Build history of the part. All positions in model axes, mm. Round coordinates to 2 decimals unless told otherwise and drop trailing zeros. Order: outer loops, then holes, each group sorted by start corner. A loop starts at its lowest first (then second) coordinate and runs counter-clockwise, first axis right, second up. Notation, with made-up numbers: M 12.5,63 L 24.5,63 A12 cw 24.5,71 Z; hole C 27,60 d5. An arc over 180 degrees is marked long. Use CSV: the item, a comma, the result in double quotes.
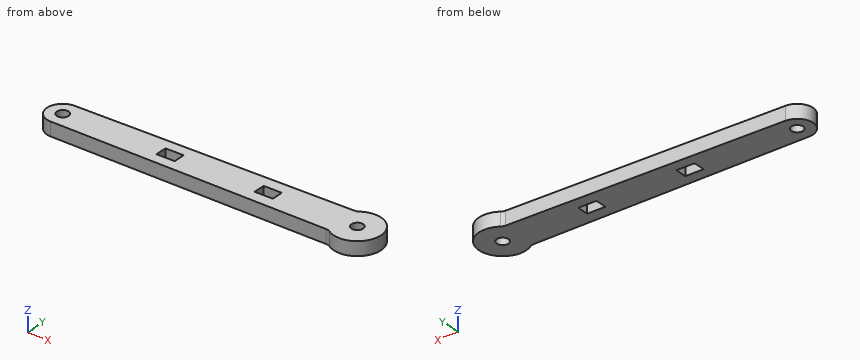
from build123d import *

# Parameters (mm, degrees)
SKETCH1_R           = 1.5
SKETCH1_W           = 4.635083662
SKETCH1_H           = 3
BOSS_EXTRUDE1_DEPTH = 3.5
FILLET1_R           = 2


with BuildPart() as part:
    # Sketch1 → Boss-Extrude1 (new body)
    with BuildSketch(Plane.XY):
        with BuildLine():
            Line((-75.039443802, 3.999805519), (-3.725751189, 4.703060501))
            ThreePointArc((-3.725751189, 4.703060501), (6, 0), (-3.725751189, -4.703060501))
            Line((-3.725751189, -4.703060501), (-75.039443802, -3.999805519))
            ThreePointArc((-75.039443802, -3.999805519), (-79, 0), (-75.039443802, 3.999805519))
        make_face()
        with Locations((-75, 0)):
            Circle(SKETCH1_R, mode=Mode.SUBTRACT)
        Circle(SKETCH1_R, mode=Mode.SUBTRACT)
        with Locations((-47.682458169, 0)):
            Rectangle(SKETCH1_W, SKETCH1_H, mode=Mode.SUBTRACT)
        with Locations((-22.682458169, 0)):
            Rectangle(SKETCH1_W, SKETCH1_H, mode=Mode.SUBTRACT)
    extrude(amount=BOSS_EXTRUDE1_DEPTH)

    # Fillet1
    fillet1_edges = [part.edges().sort_by_distance(p)[0] for p in [
        (-3.725751189, 4.703060501, 1.75),
        (-3.725751189, -4.703060501, 1.75),
    ]]
    fillet(fillet1_edges, radius=FILLET1_R)


solid = part.part
(1) Cut at B-B, the plane x = 0. Give the cut face in (y, z).
Answer block:
outline,"M -6,0 L -1.5,0 L -1.5,3.5 L -6,3.5 Z; M 1.5,0 L 6,0 L 6,3.5 L 1.5,3.5 Z"
(2) Drop flat-ended pins along their axis: pin 1 (1.8 mm diameter, centred on x = -23.5, z = 1, fed in from -Y); pin 2 (1.5 mm diameter, centred on x = -65.5, z = 2, fed in from +Y); pin 3 (2 mm diameter, centred on y = 2, z = 2.5, fed in from -X). Give the stop position or say it passes through.
Answer block:
pin 1,"stops at y = -4.52"
pin 2,"stops at y = 4.1"
pin 3,"stops at x = -78.87"
(3) Cut at C-C, the plane z = 2.6. Give the cut face in (x, y).
Answer block:
outline,"M -75.04,-4 L -4.36,-4.7 A2 cw -3.28,-5.02 A6 ccw long -3.28,5.02 A2 cw -4.36,4.7 L -75.04,4 A4 ccw Z; hole C -75,0 d3; hole M -50,-1.5 L -45.36,-1.5 L -45.36,1.5 L -50,1.5 Z; hole M -25,-1.5 L -20.36,-1.5 L -20.36,1.5 L -25,1.5 Z; hole C 0,0 d3"
(4) Cut at D-D, the plane x = -18. Give the cut face in (y, z), and give its area (3 significant figures).
Answer block:
outline,"M -4.56,0 L 4.56,0 L 4.56,3.5 L -4.56,3.5 Z"
area,"31.9 mm²"
(5) Wall check: line 1 (Y direction, x = -75, z = 2.25); line 2 (Y direction, x = 0, z = 1.6); line 3 (Y direction, x = -11.5, z = 1.5). Give the ranges that are in metal, low to high. Write a range as from..to.
Answer block:
line 1,"y = -4..-1.5, 1.5..4"
line 2,"y = -6..-1.5, 1.5..6"
line 3,"y = -4.63..4.63"
(6) Cut at A-A, the plane y = 0. Give the cut face in (x, z).
Answer block:
outline,"M -79,0 L -76.5,0 L -76.5,3.5 L -79,3.5 Z; M -73.5,0 L -50,0 L -50,3.5 L -73.5,3.5 Z; M -45.36,0 L -25,0 L -25,3.5 L -45.36,3.5 Z; M -20.36,0 L -1.5,0 L -1.5,3.5 L -20.36,3.5 Z; M 1.5,0 L 6,0 L 6,3.5 L 1.5,3.5 Z"
